Study the drawing (mm; zero at the part's minimum x, y, z) and answer. Coordinates: 2 decimals unless noted, no trailing zeros. Order: outer loops, then holes, each group sorted by start corner. A loop starts at its lowest first (then second) coordinate and runs counter-clockwise, first axis right, second up.
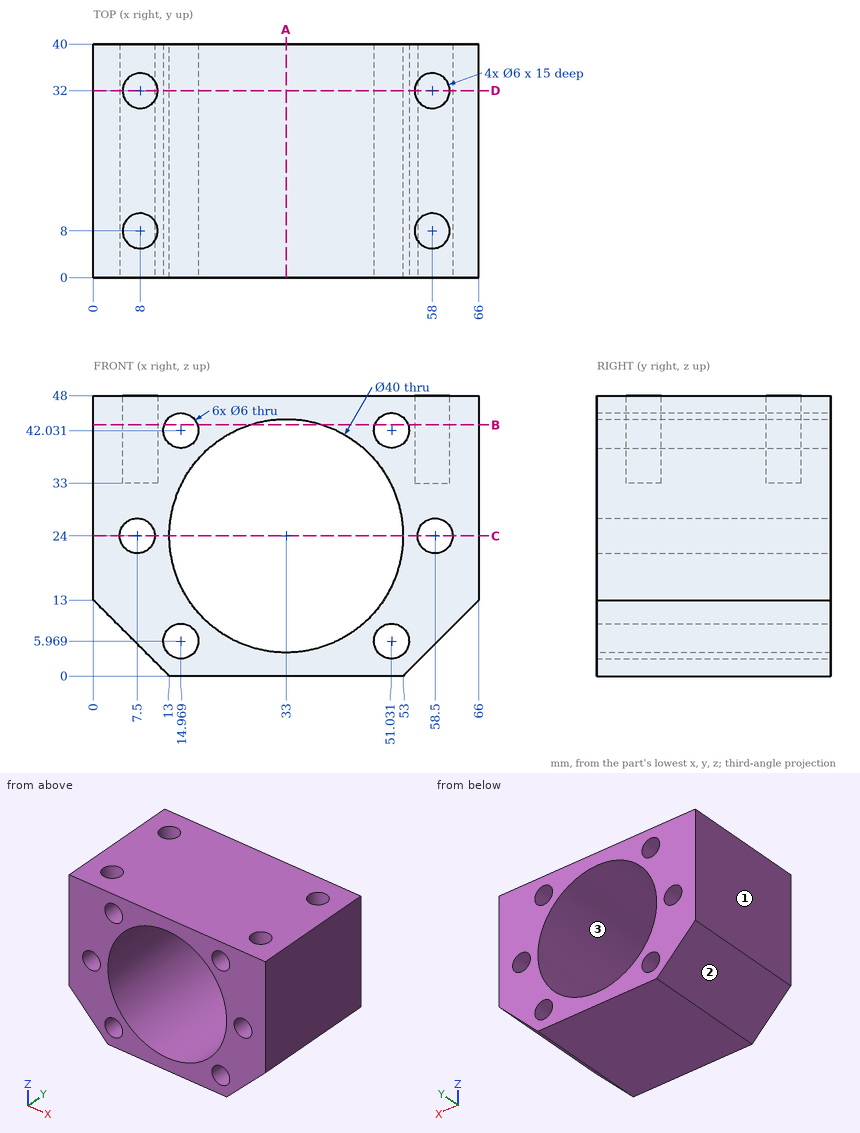
1) A cutting plane is placed at C-C, the plane z = 24. Determine the outline of the cut face in (x, y).
A:
outline: (0, 0) - (4.5, 0) - (4.5, 40) - (0, 40) - close; (10.5, 0) - (13, 0) - (13, 40) - (10.5, 40) - close; (53, 0) - (55.5, 0) - (55.5, 40) - (53, 40) - close; (61.5, 0) - (66, 0) - (66, 40) - (61.5, 40) - close
2) A cutting plane is placed at A-A, the plane x = 33. Determine the outline of the cut face in (y, z), and give its area (3 significant figures).
A:
outline: (0, 0) - (40, 0) - (40, 4) - (0, 4) - close; (0, 44) - (40, 44) - (40, 48) - (0, 48) - close
area: 320 mm2
3) Flat-ended cylindrical pins translate along their axes: pin 1 Ø4 at (y, z) = (34, 6) entering from -X; pin 2 Ø5 at (x, z) = (58.5, 24) entering from +Y; pin 3 Ø8 at (x, z) = (51.03, 5.97) entering from +Y; pin 4 Ø5.5 at (x, y) = (58, 32) entering from +Z. Find the tip coordinate at first contact, or state that the pin passes through.
A:
pin 1: stops at x = 5
pin 2: passes through
pin 3: stops at y = 40
pin 4: stops at z = 33
4) A cutting plane is placed at B-B, the plane z = 43. Determine the outline of the cut face in (x, y) (1 decimal).
A:
outline: (0, 0) - (12.1, 0) - (12.1, 40) - (0, 40) - close; (17.8, 0) - (26.8, 0) - (26.8, 40) - (17.8, 40) - close; (39.2, 0) - (48.2, 0) - (48.2, 40) - (39.2, 40) - close; (53.9, 0) - (66, 0) - (66, 40) - (53.9, 40) - close; hole circle Ø6 at (8, 8); hole circle Ø6 at (8, 32); hole circle Ø6 at (58, 8); hole circle Ø6 at (58, 32)
5) A cutting plane is placed at D-D, the plane y = 32. Determine the outline of the cut face in (x, z), and give its area (3 significant figures).
A:
outline: (0, 13) - (13, 0) - (53, 0) - (66, 13) - (66, 48) - (61, 48) - (61, 33) - (55, 33) - (55, 48) - (11, 48) - (11, 33) - (5, 33) - (5, 48) - (0, 48) - close; hole circle Ø6 at (7.5, 24); hole circle Ø6 at (14.97, 5.97); hole circle Ø6 at (14.97, 42.03); hole circle Ø40 at (33, 24); hole circle Ø6 at (51.03, 5.97); hole circle Ø6 at (51.03, 42.03); hole circle Ø6 at (58.5, 24)
area: 1,390 mm2
6) Determine the mould class of the marked faces 1, 2 and 3 for opening direction Z: pulls with the +Z half, pulls with the -Z half, needs draft (parallel to the pull), parting line crosses it, or undercut.
A:
face 1: needs draft
face 2: pulls with the -Z half
face 3: undercut
7) Straight lines are drawn through the part: line 1 (X direction, y = 29, z = 24); line 2 (Y direction, x = 58, z = 44.25); line 3 (X direction, y = 25, z = 40) (1 decimal). For each, find the intervals that lie inside material, in ascending order.
A:
line 1: x = 0 to 4.5, 10.5 to 13, 53 to 55.5, 61.5 to 66
line 2: y = 0 to 5, 11 to 29, 35 to 40
line 3: x = 0 to 12.8, 17.2 to 21, 45 to 48.8, 53.2 to 66
